Build history of the part. All positions in model axes, mm. A direction names the side the tool comes from. Coordinates: 2 decimals unless noted, no trailing zeros. Write each loop counter-clockwise with the first axis right and the second up, starting at its lowest first coordinate (ties: lowest second). Pieces come first, ordered by that corner, then holes. Notation, with made-up numbers: (82.5, 89) -> (114.5, 89) arc R34 cw to (114.5, 124) -> close; hole circle Ø6 at (17, 55). An arc over 180 degrees is marked (long way). Write each question's results on one line, items separated by ' | '. Start each with the question number.
Q1. Saw through at B-B on x = 1.75. Give the cut face in (y, z) (3 decimals).
Q2. Drop flat-ended pins along their axis: pin 1 Ø1 at (x, y) = (14.5, 10) entering from -Z; pin 2 Ø1 at (y, z) = (10.5, -3) entering from +X; pin 3 Ø1 at (y, z) = (14, -3.5) entering from +X. Give the stop position or say it passes through.
Q3. Saw through at A-A on z = 0. Count the separate pieces of the cut face and the enclosed holes in it, and give its area (3 significant figures).
Q4. Drill centre lines: line 1 (X direction, y = 2.15, z = 0); line 2 (X direction, y = 7, z = 2.5); line 3 (Z direction, x = 0.25, y = 3.25). Where is each one in solid material? Low to high.
Q5. Saw through at D-D on z = 1.5. Give the cut face in (x, y) (3 decimals).
Q6. Tool access for faces 1 (the face through (7, 0, 0)), 2 (the face through (9.9, 15.7, 1.5)): list every direction of +Z, -Z, +X, -X, +Y, -Y with a clear straight run to the whole face (end or side of a thin tool).
Q7. Two-plate mould, pull along X, no slides. Class faces 3 (the face through (-6.35, 14.09, 0.14)), 4 (the face through (15.06, 1.57, 0.31)), 5 (the face through (6, 14, -6.35)): released by +X, released by -X, zero draft, split by the parting line, or undercut.
from build123d import *

# Parameters (mm, degrees)
SKETCH1_R           = 3.2385
SKETCH1_R_2         = 3.175
BOSS_EXTRUDE1_DEPTH = 28.575
SKETCH2_R           = 3.175
SKETCH2_R_2         = 2.38125
BOSS_EXTRUDE2_DEPTH = 3.175


with BuildPart() as part:
    # Sketch1 → Boss-Extrude1 (new body)
    with BuildSketch(Plane(origin=(0, 0, 0), x_dir=(1, 0, 0), z_dir=(0, 1, 0))):
        with BuildLine():
            Line((0, 6.35), (12.7, 6.35))
            ThreePointArc((12.7, 6.35), (19.05, 0), (12.7, -6.35))
            Line((12.7, -6.35), (0, -6.35))
            ThreePointArc((0, -6.35), (-6.35, 0), (0, 6.35))
        make_face()
        with Locations(Location((0, 0, 0), (0, 0, 270))):
            Circle(SKETCH1_R, mode=Mode.SUBTRACT)
        with Locations(Location((12.7, 0, 0), (0, 0, 270))):
            Circle(SKETCH1_R_2, mode=Mode.SUBTRACT)
    extrude(amount=BOSS_EXTRUDE1_DEPTH)

    # Sketch2 → Boss-Extrude2 (add)
    with BuildSketch(Plane.XZ):
        with Locations(Location((12.7, 0, 0), (0, 0, 270))):
            Circle(SKETCH2_R)
        with Locations(Location((12.7, 0, 0), (0, 0, 270))):
            Circle(SKETCH2_R_2, mode=Mode.SUBTRACT)
    extrude(amount=-BOSS_EXTRUDE2_DEPTH)


solid = part.part
Returned:
1) outline: (0, -6.35) -> (28.575, -6.35) -> (28.575, -2.725) -> (0, -2.725) -> close; (0, 2.725) -> (28.575, 2.725) -> (28.575, 6.35) -> (0, 6.35) -> close
2) pin 1: stops at z = -6.22 | pin 2: stops at x = 18.54 | pin 3: stops at x = 18.3
3) separate pieces: 3 | enclosed holes: 0 | area: 364 mm2
4) line 1: x = -6.35 to -3.24, 3.24 to 10.32, 15.08 to 19.05 | line 2: x = -5.84 to -2.06, 2.06 to 10.74, 14.66 to 18.54 | line 3: z = -6.35 to -3.23, 3.23 to 6.35
5) outline: (-6.17, 0) -> (-2.87, 0) -> (-2.87, 28.575) -> (-6.17, 28.575) -> close; (2.87, 0) -> (10.851, 0) -> (10.851, 3.175) -> (9.902, 3.175) -> (9.902, 28.575) -> (2.87, 28.575) -> close; (14.549, 0) -> (18.87, 0) -> (18.87, 28.575) -> (15.498, 28.575) -> (15.498, 3.175) -> (14.549, 3.175) -> close
6) face 1: +Z, -Z, +X, -X, -Y | face 2: +Y
7) face 3: released by -X | face 4: undercut | face 5: zero draft
